Could you check a few things on this drawing? It's one solid part, dimensions in mm from its lowest x, y, z. Coordinates: 2 decimals unless noted, no trailing zeros. Order: outer loops, then holes, each group sorted by start corner. A loop starts at its lowest first (then second) coordinate and runs counter-clockwise, first axis right, second up. Notation, with made-up numbers: (0.25, 66) - (35.25, 66) arc R20 ccw to (35.25, 71) - close; hole circle Ø10 at (-3, -24). An arc over 180 degrees is marked (long way). Return JSON: item names as keys, results as strings. Group by question number.
1) Imagine slicing it at C-C (z = 11.5). Write out the boundary of the cut face in (x, y) (3 decimals), and give its area (3 significant figures).
2) Imagine slicing it at D-D (y = 2.3). Give the number of separate pieces and of enclosed holes in the cut face, and give its area (3 significant figures).
3) If I drill on line 1 along X through (y, z) = (0.75, 31); line 2 along X through (y, z) = (1.15, 29); line 3 along Z through (x, y) = (45, 1.85), over which ranges is the centre line in solid material (lowest first)?
4) Imagine slicing it at A-A (z = 31). Write out the boundary of the cut face in (x, y) (3 decimals).
5) Imagine slicing it at B-B (x = 45). Write out the boundary of the cut face in (y, z) (3 decimals), and give its area (3 significant figures).
6) For pin 1 Ø3 at (x, z) = (21, 15) entering from -Y; pin 2 Ø3 at (x, z) = (5, 31) entering from +Y, each with a flat end and sliding along its axis, tell me the tip position at first contact or that it passes through.
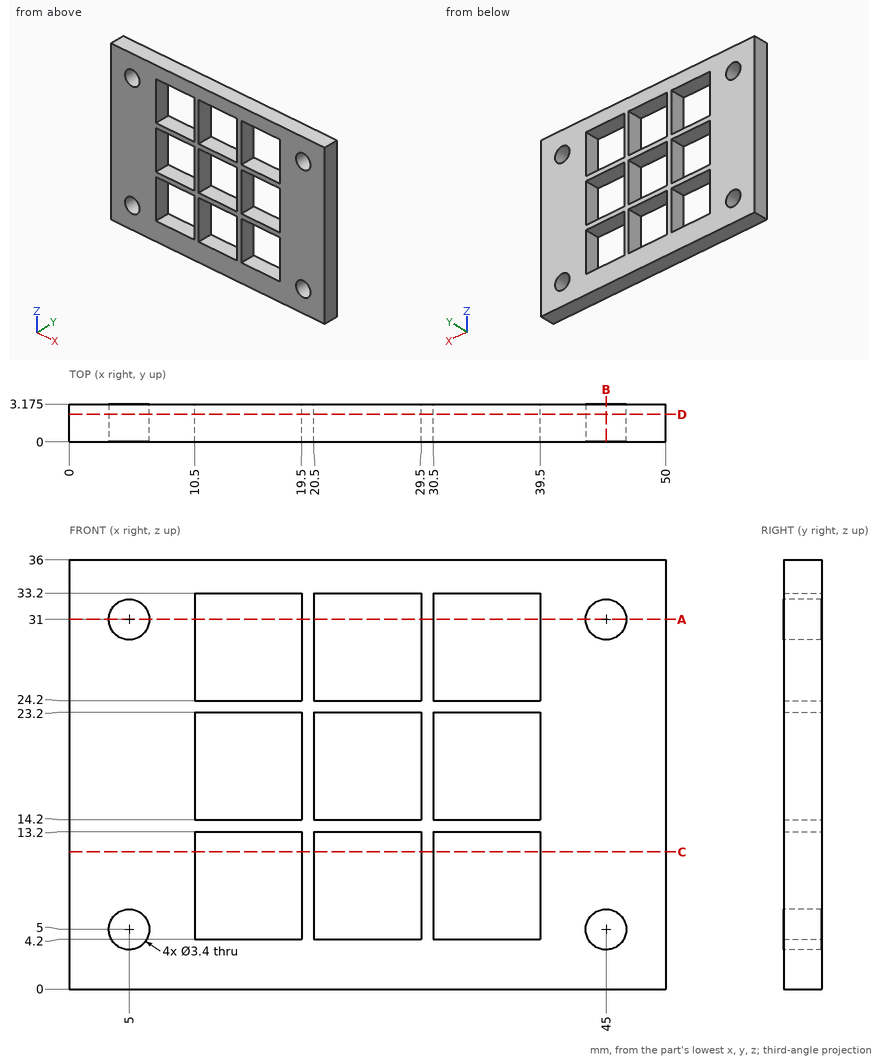
Calculated:
{
 "1": {"outline": "(0, 0) - (10.5, 0) - (10.5, 3.175) - (0, 3.175) - close; (19.5, 0) - (20.5, 0) - (20.5, 3.175) - (19.5, 3.175) - close; (29.5, 0) - (30.5, 0) - (30.5, 3.175) - (29.5, 3.175) - close; (39.5, 0) - (50, 0) - (50, 3.175) - (39.5, 3.175) - close", "area": "73.0 mm2"},
 "2": {"separate pieces": "1", "enclosed holes": "13", "area": "1,030 mm2"},
 "3": {"line 1": "0 to 3.3, 6.7 to 10.5, 19.5 to 20.5, 29.5 to 30.5, 39.5 to 43.3, 46.7 to 50", "line 2": "0 to 10.5, 19.5 to 20.5, 29.5 to 30.5, 39.5 to 50", "line 3": "0 to 3.3, 6.7 to 29.3, 32.7 to 36"},
 "4": {"outline": "(0, 0) - (3.3, 0) - (3.3, 3.175) - (0, 3.175) - close; (6.7, 0) - (10.5, 0) - (10.5, 3.175) - (6.7, 3.175) - close; (19.5, 0) - (20.5, 0) - (20.5, 3.175) - (19.5, 3.175) - close; (29.5, 0) - (30.5, 0) - (30.5, 3.175) - (29.5, 3.175) - close; (39.5, 0) - (43.3, 0) - (43.3, 3.175) - (39.5, 3.175) - close; (46.7, 0) - (50, 0) - (50, 3.175) - (46.7, 3.175) - close"},
 "5": {"outline": "(0, 0) - (3.175, 0) - (3.175, 3.3) - (0, 3.3) - close; (0, 6.7) - (3.175, 6.7) - (3.175, 29.3) - (0, 29.3) - close; (0, 32.7) - (3.175, 32.7) - (3.175, 36) - (0, 36) - close", "area": "92.7 mm2"},
 "6": {"pin 1": "y = 0", "pin 2": "through"}
}
